Can you work these out from the model? Positions are in its coordinate system, mm. Face numbers are marked on the shaded views. A direction names the side the tool comes from. Coordinates: 2 decimals unless noted, no trailing zeros. Loops run counter-clockwise (first coordinate to the right, second up) from the corner with the lowest first, then second, coordinate; pieces in that order, holes last. Notation, with made-up numbers: (80.25, 3) -> (130.25, 3) arc R35 ccw to (130.25, 40) -> close; hole circle Ø7 at (25.25, 25). An arc over 180 degrees is marked (long way). Put each result on its own line as item: value. Start each with the question number.
Item 1: If we section it at B-B on y = 12.5: Please give me the cut outline in (x, z).
Item 2: If we section it at C-C on x = -45.5: Please give me the cut outline in (y, z), plus the area to 3 significant figures.
Item 3: If we section it at A-A on y = 57: State how many separate pieces and enclosed holes the cut face has, plus the area to 3 significant figures.
Item 4: For the marked faces 1 and 2, which set-ups out of +Z, -Z, +X, -X, +Y, -Y let a thin tool reach every point of the face, with its end or its side?
Item 5: Will these pins go through, and if not, where does the flat tip stop? P1, Ø3, axis at y = 68.5, z = -69.5, coming from the +X side; P2, Ø23.5, axis at y = 28.5, z = -81, coming from the +X side; P3, Ø3, axis at x = -71, y = 68.5, coming from the +Z side.
Item 6: We'd pull the mould along X, two halves only. Please class the marked faces 3, 4 and 5: pulls with the +X half, pulls with the -X half, needs draft (parallel to the pull), parting line crosses it, or undercut.
Item 7: Please list where these lines run through material, in increasing order: L1, parallel to X at y = 15, z = 0; L2, parallel to Z at x = -10, y = 73; L3, parallel to X at y = 73, z = 0. Write a range as from..to.
Item 8: If we section it at D-D on z = 43.5: Please give me the cut outline in (x, y), plus the area to 3 significant figures.
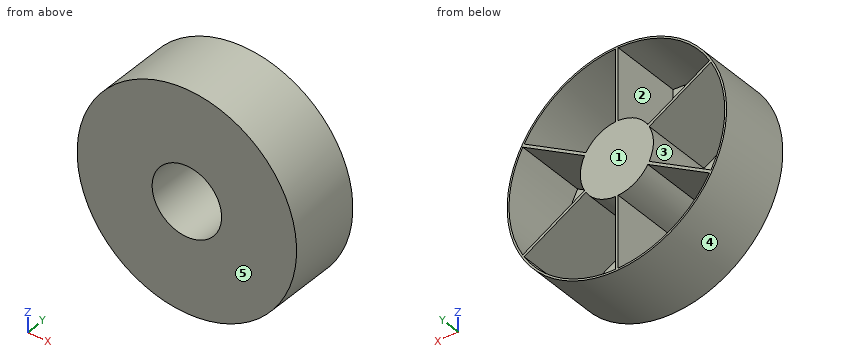
```python
from build123d import *

# Parameters (mm, degrees)
SKETCH_1_R               = 120
SKETCH_1_R_2             = 38
EXTRUDE_1_DEPTH          = 80
SHELL_1_T                = -2
EXTRUDE_START            = -78
EXTRUDE_2_DEPTH          = 78
PATTERN_CIRCULAR_1_COUNT = 6
EXTRUDE_START_2          = -8
SKETCH_3_R               = 38
EXTRUDE_3_DEPTH          = 8
SKETCH_4_R               = 5
EXTRUDE_4_DEPTH          = 24
CUT_EXTRUDE_1_DEPTH      = 19
SKETCH_6_R               = 38
SKETCH_6_R_2             = 5
CUT_EXTRUDE_2_DEPTH      = 3


with BuildPart() as part:
    # 草图1 → 凸台-拉伸1 (new body)
    with BuildSketch(Plane(origin=(0, 0, 0), x_dir=(1, 0, 0), z_dir=(0, 1, 0))):
        with Locations(Location((0, 0, 0), (0, 0, 270))):
            Circle(SKETCH_1_R)
        with Locations(Location((0, 0, 0), (0, 0, 270))):
            Circle(SKETCH_1_R_2, mode=Mode.SUBTRACT)
    extrude(amount=EXTRUDE_1_DEPTH)

    # 抽壳1
    shell_1_openings = [part.faces().sort_by_distance(p)[0] for p in [
        (0, 80, -116.60588745),
    ]]
    offset(amount=SHELL_1_T, openings=shell_1_openings, kind=Kind.INTERSECTION)

    # 草图2 → 凸台-拉伸2 (add)
    with BuildSketch(Plane(origin=(0, 80, 0), x_dir=(1, 0, 0), z_dir=(0, 1, 0)).offset(EXTRUDE_START)):
        with BuildLine():
            Line((-1.5, 117.990465717), (-1.5, 39.971865105))
            ThreePointArc((-1.5, 39.971865105), (0, 40), (1.5, 39.971865105))
            Line((1.5, 39.971865105), (1.5, 117.990465717))
            ThreePointArc((1.5, 117.990465717), (0, 118), (-1.5, 117.990465717))
        make_face()
    extrude_2 = extrude(amount=EXTRUDE_2_DEPTH)

    # 阵列(圆周)1: 凸台-拉伸2 ×6 about axis
    pattern_circular_1_axis = Axis((0, 0, 0), (0, 1, 0))
    for i in range(1, PATTERN_CIRCULAR_1_COUNT):
        add(extrude_2.rotate(pattern_circular_1_axis, i * 360 / PATTERN_CIRCULAR_1_COUNT))

    # 草图3 → 凸台-拉伸3 (add)
    with BuildSketch(Plane(origin=(0, 80, 0), x_dir=(1, 0, 0), z_dir=(0, 1, 0)).offset(EXTRUDE_START_2)):
        with Locations(Location((0, 0, 0), (0, 0, 270))):
            Circle(SKETCH_3_R)
    extrude(amount=EXTRUDE_3_DEPTH)

    # 草图4 → 凸台-拉伸4 (add)
    with BuildSketch(Plane.XZ.offset(-72)):
        with Locations(Location((0, 0, 0), (0, 0, 90))):
            Circle(SKETCH_4_R)
    extrude(amount=EXTRUDE_4_DEPTH)

    # 草图5 → 切除-拉伸1 (cut)
    with BuildSketch(Plane.XZ.offset(-48)):
        with BuildLine():
            Line((-2.049390153, 1.6), (-2.049390153, -1.6))
            ThreePointArc((-2.049390153, -1.6), (2.6, 0), (-2.049390153, 1.6))
        make_face()
    extrude(amount=-CUT_EXTRUDE_1_DEPTH, mode=Mode.SUBTRACT)

    # 草图6 → 切除-拉伸2 (cut)
    with BuildSketch(Plane.XZ.offset(-72)):
        with Locations(Location((0, 0, 0), (0, 0, 270))):
            Circle(SKETCH_6_R)
        with Locations(Location((0, 0, 0), (0, 0, 270))):
            Circle(SKETCH_6_R_2, mode=Mode.SUBTRACT)
    extrude(amount=-CUT_EXTRUDE_2_DEPTH, mode=Mode.SUBTRACT)


solid = part.part
```
Solutions:
1. outline: circle Ø240 at (0, 0); hole (-102.93, -57.7) -> (-35.37, -18.69) arc R40 cw to (-35.37, 18.69) -> (-102.93, 57.7) arc R118 ccw to start; hole (-101.43, -60.29) arc R118 ccw to (-1.5, -117.99) -> (-1.5, -39.97) arc R40 cw to (-33.87, -21.28) -> close; hole (-101.43, 60.29) -> (-33.87, 21.28) arc R40 cw to (-1.5, 39.97) -> (-1.5, 117.99) arc R118 ccw to start; hole circle Ø76 at (0, 0); hole (1.5, -117.99) arc R118 ccw to (101.43, -60.29) -> (33.87, -21.28) arc R40 cw to (1.5, -39.97) -> close; hole (1.5, 39.97) arc R40 cw to (33.87, 21.28) -> (101.43, 60.29) arc R118 ccw to (1.5, 117.99) -> close; hole (35.37, -18.69) -> (102.93, -57.7) arc R118 ccw to (102.93, 57.7) -> (35.37, 18.69) arc R40 cw to start
2. outline: (0, -111.04) -> (80, -111.04) -> (80, -108.87) -> (2, -108.87) -> (2, -28) -> (80, -28) -> (80, -24.54) -> (2, -24.54) -> (2, 24.54) -> (80, 24.54) -> (80, 28) -> (2, 28) -> (2, 108.87) -> (80, 108.87) -> (80, 111.04) -> (0, 111.04) -> close
2. area: 1,320 mm^2
3. separate pieces: 2
3. enclosed holes: 8
3. area: 3,450 mm^2
4. face 1: +Z, -Z, +X, -X, +Y
4. face 2: +Y
5. P1: x = 98.87
5. P2: x = 98
5. P3: z = 97.83
6. face 3: undercut
6. face 4: parting line crosses it
6. face 5: needs draft
7. L1: -120..-118, -40..-38, 38..40, 118..120
7. L2: -119.58..-117.58, -38.73..-36.66, 36.66..38.73, 117.58..119.58
7. L3: -120..-118, -40..-38, -5..5, 38..40, 118..120
8. outline: (-111.84, 0) -> (111.84, 0) -> (111.84, 80) -> (109.69, 80) -> (109.69, 2) -> (78.34, 2) -> (78.34, 80) -> (72.34, 80) -> (72.34, 2) -> (1.5, 2) -> (1.5, 80) -> (-1.5, 80) -> (-1.5, 2) -> (-72.34, 2) -> (-72.34, 80) -> (-78.34, 80) -> (-78.34, 2) -> (-109.69, 2) -> (-109.69, 80) -> (-111.84, 80) -> close
8. area: 1,950 mm^2
